```python
from build123d import *

# Parameters (mm, degrees)
BOSS_EXTRU_1_DEPTH = 3


with BuildPart() as part:
    # Esquisse1 → Boss.-Extru.1 (new body)
    with BuildSketch(Plane.XY):
        Polygon((-49.608259545, 25.410202795), (20.391740455, 25.410202795), (20.391740455, 21.410202795), (23.391740455, 21.410202795), (23.391740455, 17.410202795), (20.391740455, 17.410202795), (20.391740455, 13.410202795), (23.391740455, 13.410202795), (23.391740455, 9.410202795), (20.391740455, 9.410202795), (20.391740455, 5.410202795), (23.391740455, 5.410202795), (23.391740455, 1.410202795), (20.391740455, 1.410202795), (20.391740455, -2.589797205), (23.391740455, -2.589797205), (23.391740455, -6.589797205), (20.391740455, -6.589797205), (20.391740455, -10.589797205), (23.391740455, -10.589797205), (23.391740455, -14.589797205), (20.391740455, -14.589797205), (-49.608259545, -14.589797205), (-52.608259545, -14.589797205), (-52.608259545, -10.589797205), (-49.608259545, -10.589797205), (-49.608259545, -6.589797205), (-52.608259545, -6.589797205), (-52.608259545, -2.589797205), (-49.608259545, -2.589797205), (-49.608259545, 1.410202795), (-52.608259545, 1.410202795), (-52.608259545, 5.410202795), (-49.608259545, 5.410202795), (-49.608259545, 9.410202795), (-52.608259545, 9.410202795), (-52.608259545, 13.410202795), (-49.608259545, 13.410202795), (-49.608259545, 17.410202795), (-52.608259545, 17.410202795), (-52.608259545, 21.410202795), (-49.608259545, 21.410202795), align=None)
    extrude(amount=BOSS_EXTRU_1_DEPTH)


solid = part.part
```
Verification items for the finished model (mm, model axes). A direction names the side the tool comes from. Round coordinates to 2 decimals unless told otherwise and drop trailing zeros. Write each loop counter-clockwise with the first axis right and the second up, starting at its lowest first coordinate (ties: lowest second). Pieces come first, ordered by that corner, then holes. Notation, with made-up numbers: (-13, 80.25) - (21, 80.25) arc R20 ccw to (21, 119.25) - close; hole circle Ø11 at (-23.75, 11). An arc over 180 degrees is marked (long way). Answer as a JSON object with one key per item and string values. Group by question number.
Q1. Tool access check on faces 1 (the flat face through (-49.608, -1, 1)), 2 (the flat face through (-49.608, 23, 1)), 3 (the flat face through (22, 5.41, 1)), 4 (the flat face through (22, 21.41, 1)). Record the directions out of +Z, -Z, +X, -X, +Y, -Y that give a thin tool (end or side, any length) a straight path to the whole face; none if there is none.
Q2. Thickness scan on line 1 (X direction, y = 23, z = 0.9). Record the ranges inside material, lowest first.
Q3. Mould release check, pull along Y, two halves, no side actions. Record for faces 5 (the flat face through (-51, 21.41, 1)), 6 (the flat face through (-52.608, -13, 1)), 7 (the flat face through (22, 13.41, 1)): released by +Y, released by -Y, zero draft, split by the parting line, or undercut.
Q4. Section check A-A, the plane y = -8. Enter the section's corners in (x, z), plus the area to 3 significant figures.
Q5. Go/stop test with flat-tipped pins: pin 1 Ø1.5 at (y, z) = (22.5, 1.5) entering from -X; pin 2 Ø0.9 at (y, z) = (-9.5, 1.5) entering from +X; pin 3 Ø1.5 at (x, z) = (22, 1) entering from +Y. Record where each tip stops, or that it passes through.
Found:
{
 "1": {"face 1": "+Z, -Z, -X", "face 2": "+Z, -Z, -X, +Y", "face 3": "+Z, -Z, +X", "face 4": "+Z, -Z, +X, +Y"},
 "2": {"line 1": "x = -49.61 to 20.39"},
 "3": {"face 5": "released by +Y", "face 6": "zero draft", "face 7": "undercut"},
 "4": {"outline": "(-49.61, 0) - (20.39, 0) - (20.39, 3) - (-49.61, 3) - close", "area": "210 mm^2"},
 "5": {"pin 1": "stops at x = -49.61", "pin 2": "stops at x = 20.39", "pin 3": "stops at y = 21.41"}
}
